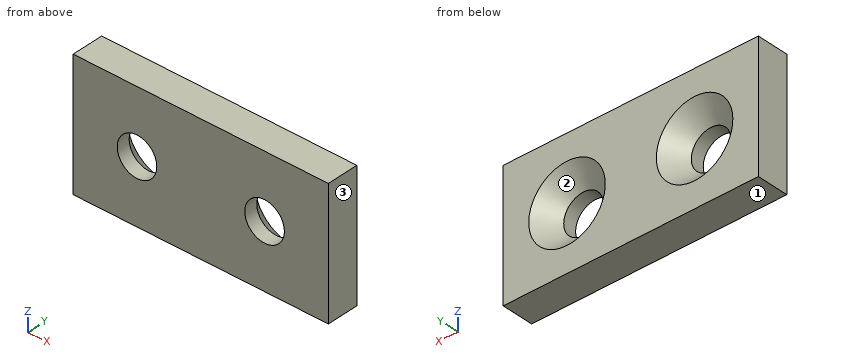
from build123d import *

# Parameters (mm, degrees)
SKETCH_1_W               = 40
SKETCH_1_H               = 20
EXTRUDE_1_DEPTH          = 5
HOLE_WIZARD_1_AT_2_COUNT = 2
HOLE_WIZARD_1_AT_2_PITCH = 20


with BuildPart() as part:
    # 草图1 → 凸台-拉伸1 (new body)
    with BuildSketch(Plane(origin=(0, 0, 0), x_dir=(1, 0, 0), z_dir=(0, 1, 0))):
        Rectangle(SKETCH_1_W, SKETCH_1_H)
    extrude(amount=EXTRUDE_1_DEPTH)

    # 草图3 → 打孔尺寸(%根据)内六角花形半沉头螺钉的类型1 (revolve, cut)
    with BuildSketch(Plane(origin=(-10, 5, 0), x_dir=(0, 0, 1), z_dir=(1, 0, 0))):
        Polygon((0, 0), (0, 5), (3.1, 5), (3.1, 2.9), (6, 0), align=None)
    hole_wizard_1 = revolve(axis=Axis((-10, 11.35, 0), (0, -1, 0)), mode=Mode.SUBTRACT)

    # 打孔尺寸(%根据)内六角花形半沉头螺钉的类型1 at 2: 打孔尺寸(%根据)内六角花形半沉头螺钉的类型1 ×2
    with Locations(*[(i * HOLE_WIZARD_1_AT_2_PITCH, 0, 0) for i in range(1, HOLE_WIZARD_1_AT_2_COUNT)]):
        add(hole_wizard_1, mode=Mode.SUBTRACT)


solid = part.part
The listing builds one solid part. Answer for the finished solid, in the listing's coordinates (mm). Face numbers are marked on the shaded views. Coordinates: 2 decimals unless noted, no trailing zeros. Loops run counter-clockwise (first coordinate to the right, second up) from the corner with the lowest first, then second, coordinate; pieces in that order, holes last.
1) Flat-ended cylindrical pins translate along their axes: pin 1 Ø5 at (x, z) = (10, 0) entering from -Y; pin 2 Ø10 at (x, z) = (-10, 0) entering from +Y. Find the tip coordinate at first contact, or state that the pin passes through.
2) Find section A-A on x = -10. Write down the section's boundary in (y, z).
3) Find the intervals of material crossed by L1, parallel to X at y = 0.5, z = 0; L2, parallel to Z at x = 10, y = 1.25; L3, parallel to Z at x = 12, y = 1.2, in increasing order.
4) Find section C-C on y = 1.5. Write down the section's boundary in (x, z), then the cut area to 3 significant figures.
5) Find section D-D on y = 3.25. Write down the section's boundary in (x, z), then the cut area to 3 significant figures.
6) Determine the mould class of the marked faces 1, 2 and 3 for opening direction X: pulls with the +X half, pulls with the -X half, needs draft (parallel to the pull), parting line crosses it, or undercut.
7) Find section B-B on z = 0. Write down the section's boundary in (x, y).
Values:
1. pin 1: passes through
1. pin 2: stops at y = 4
2. outline: (0, -10) - (5, -10) - (5, -6) - (2.1, -3.1) - (0, -3.1) - close; (0, 3.1) - (2.1, 3.1) - (5, 6) - (5, 10) - (0, 10) - close
3. L1: x = -20 to -13.1, -6.9 to 6.9, 13.1 to 20
3. L2: z = -10 to -3.1, 3.1 to 10
3. L3: z = -10 to -2.37, 2.37 to 10
4. outline: (-20, -10) - (20, -10) - (20, 10) - (-20, 10) - close; hole circle Ø6.2 at (-10, 0); hole circle Ø6.2 at (10, 0)
4. area: 740 mm2
5. outline: (-20, -10) - (20, -10) - (20, 10) - (-20, 10) - close; hole circle Ø8.5 at (-10, 0); hole circle Ø8.5 at (10, 0)
5. area: 687 mm2
6. face 1: needs draft
6. face 2: undercut
6. face 3: pulls with the +X half
7. outline: (-20, 0) - (-13.1, 0) - (-13.1, 2.1) - (-16, 5) - (-20, 5) - close; (-6.9, 0) - (6.9, 0) - (6.9, 2.1) - (4, 5) - (-4, 5) - (-6.9, 2.1) - close; (13.1, 0) - (20, 0) - (20, 5) - (16, 5) - (13.1, 2.1) - close
